Design review of the part built by this model. Coordinates are the model's own, in mm. A direction names the side the tool comes from. Coordinates: 2 decimals unless noted, no trailing zeros. Order: outer loops, then holes, each group sorted by start corner. A loop starts at its lowest first (then second) coordinate and runs counter-clockwise, first axis right, second up. Notation, with made-up numbers: (21, 52.5) -> (43, 52.5) arc R16 cw to (43, 60.5) -> close; hole circle Ø5 at (-9, 85.5). An arc over 180 degrees is marked (long way). Write item = value, one per line.
```python
from build123d import *

# Parameters (mm, degrees)
F1_DEPTH = 43.7
F2_R     = 6
F3_R     = 1
F4_R     = 0.5


with BuildPart() as f1:
    # F0 (on Front) → F1 (new body)
    with BuildSketch(Plane.XZ):
        Polygon((-17.729146, 0), (17.770854, 0), (96.619631, 36.767789), (95.351776, 39.486712), (17.10577, 3), (-17.064062, 3), (-95.310069, 39.486712), (-96.577924, 36.767789), align=None)
    extrude(amount=F1_DEPTH)

    # F2
    f2_edges = [f1.edges().sort_by_distance(p)[0] for p in [
        (-95.943996, -43.7, 38.12725),
        (-95.943996, 0, 38.12725),
        (95.985704, 0, 38.12725),
        (95.985704, -43.7, 38.12725),
    ]]
    fillet(f2_edges, radius=F2_R)

    # F3
    f3_edges = [f1.edges().sort_by_distance(p)[0] for p in [
        (17.770854, -21.85, 0),
        (-17.729146, -21.85, 0),
        (17.10577, -21.85, 3),
        (-17.064062, -21.85, 3),
    ]]
    fillet(f3_edges, radius=F3_R)

    # F4
    f4_edges = [f1.edges().sort_by_distance(p)[0] for p in [
        (-53.568604, 0, 20.022347),
        (0.020854, 0, 3),
        (-54.535074, 0, 17.162886),
        (-17.93007, -21.85, 0.093692),
        (-94.985215, -1.757359, 36.025097),
        (-54.535074, -43.7, 17.162886),
        (-96.577924, -21.85, 36.767789),
        (-94.985215, -41.942641, 36.025097),
    ]]
    fillet(f4_edges, radius=F4_R)


solid = f1.part
```
(1) We need section A-A (y = -19.5). Write out the cut boundary in (x, z).
Report:
outline = (-96.37, 37.22) arc R0.5 ccw to (-96.12, 36.56) -> (-17.93, 0.09) arc R1 ccw to (-17.51, 0) -> (17.55, 0) arc R1 ccw to (17.97, 0.09) -> (96.17, 36.56) arc R0.5 ccw to (96.41, 37.22) -> (95.56, 39.03) arc R0.5 ccw to (94.9, 39.28) -> (17.31, 3.09) arc R1 cw to (16.88, 3) -> (-16.84, 3) arc R1 cw to (-17.26, 3.09) -> (-94.86, 39.28) arc R0.5 ccw to (-95.52, 39.03) -> close
(2) We need section B-B (x = 8.5). Write out the cut boundary in (y, z).
Report:
outline = (-43.7, 0.5) arc R0.5 ccw to (-43.2, 0) -> (-0.5, 0) arc R0.5 ccw to (0, 0.5) -> (0, 2.5) arc R0.5 ccw to (-0.5, 3) -> (-43.2, 3) arc R0.5 ccw to (-43.7, 2.5) -> close
(3) For faces 1 (the cylindrical face through (53.17, -0.14, 19.65)), 2 (the cylindrical face through (54.18, -43.56, 20.12)), 3 (the flat face through (0, -22, 3)), list the 3-axis set-ups (+Z, -Z, +X, -X, +Y, -Y) from which the entire face can be reached by the end or side of a thin tool; tool diameter is ignored.
Report:
face_1 = +Z, +Y
face_2 = +Z, -Y
face_3 = +Z, +Y, -Y
(4) Insertion check: pin 1 (4 mm diameter, centred on y = -19, z = 24.5, fed in from -X); pin 2 (4 mm diameter, centred on y = -11, z = 29, fed in from -X); pin 3 (4 mm diameter, centred on x = -73, y = -6, fed in from -Z). Each pin has a flat end and moves straight along its axis. Give the tip position at first contact, or say it passes through.
Report:
pin_1 = -74.56
pin_2 = -84.21
pin_3 = 24.84
(5) For L1, parallel to Z at x = 15.5, y = -34.5; L2, parallel to X at y = -6.5, z = 13.5; L3, parallel to X at y = -37.5, z = 28.5, list the stretches that pass through material, from the lowest coordinate up.
Report:
L1 = 0 to 3
L2 = -46.68 to -39.58, 39.62 to 46.72
L3 = -78.85 to -71.75, 71.79 to 78.89
(6) The part is to be moulded in two halves that separate along X. For faces 4 (the cylindrical face through (-54.98, -43.56, 17.54)), 5 (the cylindrical face through (-53.124, -43.557, 19.649)), 6 (the cylindrical face through (94.429, -41.896, 37.417)), say which applies: released by +X, released by -X, zero draft, split by the parting line, or undercut.
Report:
face_4 = released by -X
face_5 = undercut
face_6 = released by +X
